Input: part model. Units: mm. Frame: model coordinates. Face numbers are marked on the shaded views. A direction names the side the tool comes from. Give positions to 0.01 mm unless a question says otherwise; leave off trailing zeros. Order: outer loops, then holes, each group sorted by start corner. A loop starts at its lowest first (then second) coordinate and runs counter-clockwise, first axis right, second up. Notation, with made-up numbers: (22, 46.5) - (33, 46.5) arc R21 ccw to (33, 57.5) - close; hole circle Ø3 at (81, -12). An arc over 180 degrees is marked (long way). Use a Markdown table: item, result.
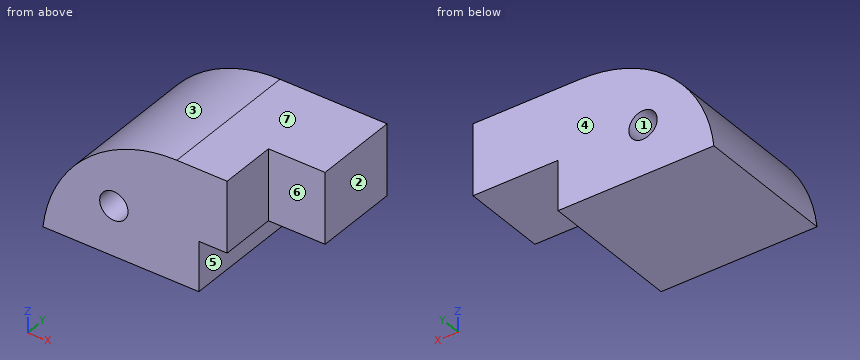
from build123d import *

# Parameters (mm, degrees)
F0_W         = 215.9
F0_H         = 127
F1_DEPTH     = 82.55
F2_W         = 76.2
F2_H         = 44.45
F3_DEPTH     = 127.001
F4_W         = 50.8
F4_H         = 37.5581905246
F5_DEPTH     = 82.551
F6_R         = 7.8160058593
F7_DEPTH     = 0.254
F8_R         = 12.7
F9_DEPTH     = 127.001
F10_T1_DEPTH = 699.3812649799
F11_DEPTH    = 107.95
F14_W        = 76.2
F14_H        = 44.45
F15_DEPTH    = 127.001
F13_W        = 50.8
F13_H        = 63.5
F16_DEPTH    = 50.8
F17_R        = 12.7
F18_DEPTH    = 127.001
F19_T1_DEPTH = 726.8985851792


# Not quite as in the source:
# - a fillet or chamfer that OpenCascade refuses, or shapes differently, is made with other operations: its cross-section is extruded or revolved along the edge and cut away or added


with BuildPart() as f1:
    # F0 (on Top) → F1 (new body)
    with BuildSketch(Plane.XY):
        with Locations((13.1497114167, 63.5)):
            Rectangle(F0_W, F0_H)
    extrude(amount=F1_DEPTH)

    # F2 (on face) → F3 (cut, through all)
    with BuildSketch(Plane(origin=(0, 127, 0), x_dir=(-1, 0, 0), z_dir=(0, 1, 0))):
        with Locations((-82.9997114167, 22.225)):
            Rectangle(F2_W, F2_H)
    extrude(amount=-F3_DEPTH, mode=Mode.SUBTRACT)

    # F4 (on face) → F5 (cut, through all)
    with BuildSketch(Plane.XY.offset(82.55)):
        with Locations((95.6997114167, 18.7790952623)):
            Rectangle(F4_W, F4_H)
    extrude(amount=-F5_DEPTH, mode=Mode.SUBTRACT)

    # F6 (on face) → F7 (cut)
    with BuildSketch(Plane.YZ.offset(121.0997114167)):
        with Locations((84.554515779, 63.2054284215)):
            Circle(F6_R)
    extrude(amount=-F7_DEPTH, mode=Mode.SUBTRACT)

    # F8 (on face) → F9 (cut, through all)
    with BuildSketch(Plane(origin=(0, 127, 0), x_dir=(-1, 0, 0), z_dir=(0, 1, 0))):
        with Locations((31.3002885833, 44.45)):
            Circle(F8_R)
    extrude(amount=-F9_DEPTH, mode=Mode.SUBTRACT)

    # F10: fillet of radius 120.65 on 1 edges, made by hand

    # F10_s2 → F10_t1 (cut)
    with BuildSketch(Plane.XZ.offset(-413.19063249)):
        with BuildLine():
            ThreePointArc((-94.8002885833, 0), (-50.8919372849, 59.7600722971), (19.6759644126, 82.55))
            Line((19.6759644126, 82.55), (19.6759644126, 84.963))
            Line((19.6759644126, 84.963), (-94.8002885833, 84.963))
            Line((-94.8002885833, 84.963), (-97.2132885833, 82.55))
            ThreePointArc((-97.2132885833, 82.55), (-97.2132885833, 41.275), (-97.0898136433, 0.762))
            Line((-97.0898136433, 0.762), (-94.8002885833, 0))
        make_face()
    extrude(amount=F10_T1_DEPTH, mode=Mode.SUBTRACT)

    # F0 (on Top) → F11 (join)
    with BuildSketch(Plane.XY):
        with Locations((13.1497114167, 63.5)):
            Rectangle(F0_W, F0_H)
    extrude(amount=F11_DEPTH)

    # F14 (on face) → F15 (cut, through all)
    with BuildSketch(Plane(origin=(0, 127, 0), x_dir=(-1, 0, 0), z_dir=(0, 1, 0))):
        with Locations((-82.9997114167, 22.225)):
            Rectangle(F14_W, F14_H)
    extrude(amount=-F15_DEPTH, mode=Mode.SUBTRACT)

    # F13 (on face) → F16 (cut)
    with BuildSketch(Plane.YZ.offset(121.0997114167)):
        with Locations((25.4, 76.2)):
            Rectangle(F13_W, F13_H)
    extrude(amount=-F16_DEPTH, mode=Mode.SUBTRACT)

    # F17 (on face) → F18 (cut, through all)
    with BuildSketch(Plane(origin=(0, 127, 0), x_dir=(-1, 0, 0), z_dir=(0, 1, 0))):
        with Locations((31.3002885833, 44.45)):
            Circle(F17_R)
    extrude(amount=-F18_DEPTH, mode=Mode.SUBTRACT)

    # F19: fillet of radius 120.65 on 1 edges, made by hand

    # F19_s2 → F19_t1 (cut)
    with BuildSketch(Plane.XZ.offset(-426.9492925896)):
        with BuildLine():
            ThreePointArc((-94.8002885833, 0), (-55.5180544698, 76.9902377631), (25.1794284525, 107.95))
            Line((25.1794284525, 107.95), (-94.8002885833, 107.95))
            Line((-94.8002885833, 107.95), (-94.8002885833, 0))
        make_face()
    extrude(amount=F19_T1_DEPTH, mode=Mode.SUBTRACT)


solid = f1.part
1. Mould query, pull axis X, two halves, no side actions, for the marked faces 1, 2, 3 and 4. Classes: pulls with the +X half, pulls with the -X half, needs draft (parallel to the pull), parting line crosses it, or undercut.
Response:
| item | result |
|---|---|
| face 1 | undercut |
| face 2 | pulls with the +X half |
| face 3 | pulls with the -X half |
| face 4 | needs draft |
2. Material intervals for line 1 along Y through (x, z) = (82, 89.5); line 2 along Z through (x, y) = (92, 57.5); line 3 along X through (y, z) = (118, 53), sorted ascending.
Response:
| item | result |
|---|---|
| line 1 | y = 50.8 to 127 |
| line 2 | z = 44.45 to 107.95 |
| line 3 | x = -76.01 to -40.69, -21.91 to 121.1 |
3. Section query C-C (z = 68). Return loops of the section in (x, y), then the cut area to 3 significant figures.
Response:
| item | result |
|---|---|
| outline | (-64.51, 0) - (70.3, 0) - (70.3, 50.8) - (121.1, 50.8) - (121.1, 127) - (-64.51, 127) - close |
| area | 21,000 mm^2 |
4. Section query A-A (y = 81). Return loops of the section in (x, z).
Response:
| item | result |
|---|---|
| outline | (-94.8, 0) - (44.9, 0) - (44.9, 44.45) - (121.1, 44.45) - (121.1, 107.95) - (25.18, 107.95) arc R120.65 ccw to start; hole circle Ø25.4 at (-31.3, 44.45) |
5. Pin query (flat end, axial travel): pin 1 (2 mm diameter, centred on y = 70.5, z = 11, fed in from +X); pin 2 (1.5 mm diameter, centred on y = 70, z = 39.5, fed in from -X); pin 3 (4 mm diameter, centred on y = 24, z = 47.5, fed in from -X). Return the tip coordinate at first contact, or that it passes through.
Response:
| item | result |
|---|---|
| pin 1 | stops at x = 44.9 |
| pin 2 | stops at x = -83.95 |
| pin 3 | stops at x = -80.5 |
6. Set-up query: the marked faces 5, 6 and 7. Return all of +Z, -Z, +X, -X, +Y, -Y with unobstructed straight access to the full face (end or side cutting, diameter ignored); none if empty.
Response:
| item | result |
|---|---|
| face 5 | -Z, +X, +Y, -Y |
| face 6 | +Z, -Z, +X, -Y |
| face 7 | +Z, +X, -X, +Y, -Y |
7. Section query D-D (z = 98). Return loops of the section in (x, y), then the cut area to 3 significant figures.
Response:
| item | result |
|---|---|
| outline | (-22.8, 0) - (70.3, 0) - (70.3, 50.8) - (121.1, 50.8) - (121.1, 127) - (-22.8, 127) - close |
| area | 15,700 mm^2 |
8. Section query B-B (x = 72.5). Return loops of the section in (y, z), then the cut area to 3 significant figures.
Response:
| item | result |
|---|---|
| outline | (50.8, 44.45) - (127, 44.45) - (127, 107.95) - (50.8, 107.95) - close |
| area | 4,840 mm^2 |
